Part model, mm, in its own coordinate system. Coordinates: 2 decimals unless noted, no trailing zeros. Loops run counter-clockwise (first coordinate to the right, second up) from the corner with the lowest first, then second, coordinate; pieces in that order, holes last. Notation, with made-up numbers: (-32, 54.25) -> (-24, 54.25) arc R31 cw to (-24, 87.25) -> close; hole circle Ø10 at (-34.75, -33.75). An arc over 180 degrees is marked (long way). One line per item, written item: value. Start each with the question number.
Autodesk Inventor part; units mm, degrees
ref_plane "YZ Plane" through (0, 0, 0) normal (1, 0, 0) x (0, 1, 0)
ref_plane "XZ Plane" through (0, 0, 0) normal (0, 1, 0) x (-1, 0, 0)
ref_plane "XY Plane" through (0, 0, 0) normal (0, 0, 1) x (1, 0, 0)
sketch "Sketch1" plane through (0, 0, 0) normal (0, 1, 0) x (-1, 0, 0)
  line L0 (66, 0) -> (-66, 0) construction
  line L1 (66, 9) -> (-66, 9)
  line L2 (-66, -9) -> (66, -9)
  arc A0 (66, -9) -> (66, 9) centre (66, 0) ccw
  arc A1 (-66, 9) -> (-66, -9) centre (-66, 0) ccw
  point P0 (0, 0)
  dimension "d0" = 66
  dimension "d1" = 18
extrude "Extrusion1" add sketch "Sketch1" along normal blind 1.3
sketch "Sketch2" plane through (0, 1.3, 0) normal (0, 1, 0) x (1, 0, 0)
  arc A0 (-66, 9) -> (-66, -9) centre (-66, 0) ccw
  arc A1 (66, -9) -> (66, 9) centre (66, 0) ccw
  point P0 (0, 0)
hole "Hole1" at (-66, 1.3, 0) at (66, 1.3, 0) direction (0, -1, 0) diameter 3 end through all
thread "Thread1"
thread "Thread2"
properties part number "upper link"
1) Slice it at A-A (z = 0). Give the cut face in (x, y).
2) Slice it at C-C (z = 5.5). Give the cut face in (x, y).
3) Probe line 1 (X direction, y = 0.45, z = 0); line 2 (X direction, y = 0.65, z = 0.5); line 3 (Z direction, x = -66, y = 0.6). List the from-to ranges inside material, lowest first. Write a range as from..to.
4) Slice it at B-B (y = 0.25). Give the cut face in (x, z).
Check sheet entries:
1. outline: (-75, 0) -> (-67.5, 0) -> (-67.5, 1.3) -> (-75, 1.3) -> close; (-64.5, 0) -> (64.5, 0) -> (64.5, 1.3) -> (-64.5, 1.3) -> close; (67.5, 0) -> (75, 0) -> (75, 1.3) -> (67.5, 1.3) -> close
2. outline: (-73.12, 0) -> (73.12, 0) -> (73.12, 1.3) -> (-73.12, 1.3) -> close
3. line 1: x = -75..-67.5, -64.5..64.5, 67.5..75
3. line 2: x = -74.99..-67.41, -64.59..64.59, 67.41..74.99
3. line 3: z = -9..-1.5, 1.5..9
4. outline: (-66, -9) -> (66, -9) arc R9 ccw to (66, 9) -> (-66, 9) arc R9 ccw to start; hole circle Ø3 at (-66, 0); hole circle Ø3 at (66, 0)
